Work out the finished part from the listing and answer in its coordinate system (mm). Round coordinates to 2 decimals unless told otherwise and drop trailing zeros. Order: outer loops, then holes, each group sorted by start corner. A loop starts at its lowest first (then second) coordinate and runs counter-clockwise, first axis right, second up. Notation, with made-up numbers: (57, 58) -> (83, 58) arc R21 ccw to (83, 62) -> close; hole circle Ø5 at (-1.5, 24.5). An arc over 180 degrees is marked (long way). Use one line per item in the form item = value.
```python
from build123d import *

# Parameters (mm, degrees)
SKETCH1_W           = 84.7
SKETCH1_H           = 44.8
BOSS_EXTRUDE1_DEPTH = 10.22
SKETCH2_W           = 24.5
SKETCH2_H           = 16.3
BOSS_EXTRUDE2_DEPTH = 2
SKETCH3_W           = 5.34
SKETCH3_H           = 9.1
SKETCH3_H_2         = 11.9
SKETCH3_H_3         = 11.1
SKETCH3_H_4         = 15.17
SKETCH3_H_5         = 17.32
SKETCH3_H_6         = 8
SKETCH3_H_7         = 13
SKETCH3_H_8         = 17.2
CUT_EXTRUDE1_DEPTH  = 2
SKETCH4_R           = 1.25
CUT_EXTRUDE2_DEPTH  = 50.443006583
SKETCH5_R           = 2
CUT_EXTRUDE3_DEPTH  = 1
SKETCH7_W           = 8.64
SKETCH7_H           = 3.2
CUT_EXTRUDE5_DEPTH  = 2
SKETCH8_W           = 5
SKETCH8_H           = 2
CUT_EXTRUDE6_DEPTH  = 2
SKETCH9_W           = 20.33
SKETCH9_H           = 3.1
SKETCH9_W_2         = 5.5
SKETCH9_H_2         = 2
CUT_EXTRUDE7_DEPTH  = 2
SKETCH10_W          = 13.9
SKETCH10_H          = 2.2
CUT_EXTRUDE8_DEPTH  = 2
CUT_EXTRUDE9_DEPTH  = 0.1


with BuildPart() as part:
    # Sketch1 → Boss-Extrude1 (new body)
    with BuildSketch(Plane(origin=(0, 0, 0), x_dir=(1, 0, 0), z_dir=(0, 1, 0))):
        Rectangle(SKETCH1_W, SKETCH1_H)
    extrude(amount=BOSS_EXTRUDE1_DEPTH)

    # Sketch2 → Boss-Extrude2 (add)
    with BuildSketch(Plane(origin=(0, 10.22, 0), x_dir=(1, 0, 0), z_dir=(0, 1, 0))):
        with Locations((-30.1, 0)):
            Rectangle(SKETCH2_W, SKETCH2_H)
    extrude(amount=BOSS_EXTRUDE2_DEPTH)

    # Sketch3 → Cut-Extrude1 (cut)
    with BuildSketch(Plane(origin=(0, 10.22, 0), x_dir=(1, 0, 0), z_dir=(0, 1, 0))):
        with Locations((-2.92, -15.5)):
            Rectangle(SKETCH3_W, SKETCH3_H)
        with Locations((-2.92, -1.82)):
            Rectangle(SKETCH3_W, SKETCH3_H_2)
        with Locations((-2.92, 13.95)):
            Rectangle(SKETCH3_W, SKETCH3_H_2)
        with Locations((5.22, 14.35)):
            Rectangle(SKETCH3_W, SKETCH3_H_3)
        with Locations((5.22, -1.82)):
            Rectangle(SKETCH3_W, SKETCH3_H_2)
        with Locations((5.22, -15.5)):
            Rectangle(SKETCH3_W, SKETCH3_H)
        with Locations((13.46, -15.5)):
            Rectangle(SKETCH3_W, SKETCH3_H)
        with Locations((13.46, -3.22)):
            Rectangle(SKETCH3_W, SKETCH3_H)
        with Locations((13.46, 12.315)):
            Rectangle(SKETCH3_W, SKETCH3_H_4)
        with Locations((21.6, 11.24)):
            Rectangle(SKETCH3_W, SKETCH3_H_5)
        with Locations((21.6, -4.84)):
            Rectangle(SKETCH3_W, SKETCH3_H_6)
        with Locations((21.6, -16.05)):
            Rectangle(SKETCH3_W, SKETCH3_H_6)
        with Locations((29.24, 0.8)):
            Rectangle(SKETCH3_W, SKETCH3_H_7)
        with Locations((36.88, 11.3)):
            Rectangle(SKETCH3_W, SKETCH3_H_8)
        with Locations((36.88, -11.45)):
            Rectangle(SKETCH3_W, SKETCH3_H_8)
        with Locations((-37.74, -14.1)):
            Rectangle(SKETCH3_W, SKETCH3_H_2)
        with Locations((-23.15, -14.1)):
            Rectangle(SKETCH3_W, SKETCH3_H_2)
    extrude(amount=-CUT_EXTRUDE1_DEPTH, mode=Mode.SUBTRACT)

    # Sketch4 → Cut-Extrude2 (cut, through all)
    with BuildSketch(Plane.XZ):
        with Locations(Location((-30.35, 15.75, 0), (0, 0, 270))):
            Circle(SKETCH4_R)
        with Locations(Location((-30.35, -15.75, 0), (0, 0, 270))):
            Circle(SKETCH4_R)
        with Locations(Location((31.25, 15.75, 0), (0, 0, 270))):
            Circle(SKETCH4_R)
        with Locations(Location((31.25, -15.75, 0), (0, 0, 270))):
            Circle(SKETCH4_R)
    extrude(amount=-CUT_EXTRUDE2_DEPTH, mode=Mode.SUBTRACT)

    # Sketch5 → Cut-Extrude3 (cut)
    with BuildSketch(Plane(origin=(0, 10.22, 0), x_dir=(1, 0, 0), z_dir=(0, 1, 0))):
        with Locations(Location((-30.35, -15.75, 0), (0, 0, 270))):
            Circle(SKETCH5_R)
        with Locations(Location((31.25, 15.75, 0), (0, 0, 270))):
            Circle(SKETCH5_R)
        with Locations(Location((31.25, -15.75, 0), (0, 0, 270))):
            Circle(SKETCH5_R)
        with Locations(Location((-30.35, 15.75, 0), (0, 0, 270))):
            Circle(SKETCH5_R)
    extrude(amount=-CUT_EXTRUDE3_DEPTH, mode=Mode.SUBTRACT)

    # Sketch7 → Cut-Extrude5 (cut)
    with BuildSketch(Plane.XY.offset(22.4)):
        with Locations((-11.48, 6.52)):
            Rectangle(SKETCH7_W, SKETCH7_H)
    extrude(amount=-CUT_EXTRUDE5_DEPTH, mode=Mode.SUBTRACT)

    # Sketch8 → Cut-Extrude6 (cut)
    with BuildSketch(Plane.XY.offset(22.4)):
        with Locations((23.75, 3.72)):
            Rectangle(SKETCH8_W, SKETCH8_H)
    extrude(amount=-CUT_EXTRUDE6_DEPTH, mode=Mode.SUBTRACT)

    # Sketch9 → Cut-Extrude7 (cut)
    with BuildSketch(Plane(origin=(0, 0, -22.4), x_dir=(-1, 0, 0), z_dir=(0, 0, -1))):
        with Locations((-2.885, 3.3)):
            Rectangle(SKETCH9_W, SKETCH9_H)
        with Locations((-23.2, 3.72)):
            Rectangle(SKETCH9_W_2, SKETCH9_H_2)
    extrude(amount=-CUT_EXTRUDE7_DEPTH, mode=Mode.SUBTRACT)

    # Sketch10 → Cut-Extrude8 (cut)
    with BuildSketch(Plane(origin=(42.35, 0, 0), x_dir=(0, 0, -1), z_dir=(1, 0, 0))):
        with Locations((-1.25, 3.66)):
            Rectangle(SKETCH10_W, SKETCH10_H)
    extrude(amount=-CUT_EXTRUDE8_DEPTH, mode=Mode.SUBTRACT)

    # Sketch11 → Cut-Extrude9 (cut)
    with BuildSketch(Plane(origin=(0, 12.22, 0), x_dir=(1, 0, 0), z_dir=(0, 1, 0))):
        with BuildLine():
            Line((-36.282417149, 0), (-26.882417149, 2.15))
            Line((-26.882417149, 2.15), (-27.617159632, 1.392199815))
            ThreePointArc((-27.617159632, 1.392199815), (-28.181269776, 0), (-27.617159632, -1.392199815))
            Line((-27.617159632, -1.392199815), (-26.882417149, -2.15))
            Line((-26.882417149, -2.15), (-36.282417149, 0))
        make_face()
    extrude(amount=-CUT_EXTRUDE9_DEPTH, mode=Mode.SUBTRACT)


solid = part.part
```
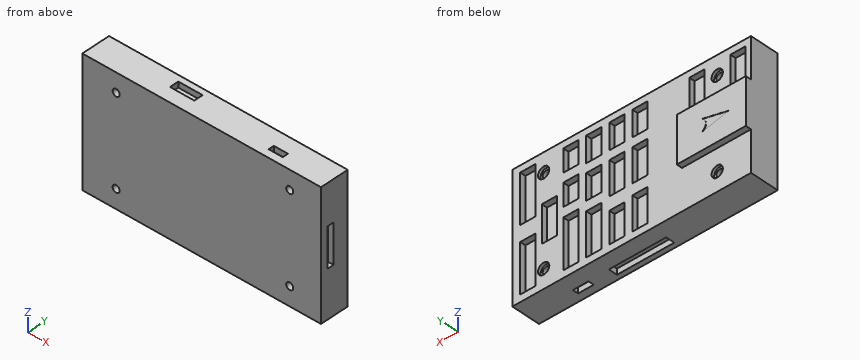
Item 1: The part is cut by section D-D, the plane x = -8.5. Give the vertices of the cut face in (y, z).
Findings:
outline = (0, -22.4) -> (10.22, -22.4) -> (10.22, 22.4) -> (8.12, 22.4) -> (8.12, 20.4) -> (4.92, 20.4) -> (4.92, 22.4) -> (0, 22.4) -> close
Item 2: The part is cut by section B-B, the plane x = -30.35. Give the vertices of the cut face in (y, z), and give its area (3 significant figures).
Findings:
outline = (0, -22.4) -> (10.22, -22.4) -> (10.22, -17.75) -> (9.22, -17.75) -> (9.22, -17) -> (0, -17) -> close; (0, -14.5) -> (9.22, -14.5) -> (9.22, -13.75) -> (10.22, -13.75) -> (10.22, -8.15) -> (12.22, -8.15) -> (12.22, -1.36) -> (12.12, -1.36) -> (12.12, 1.36) -> (12.22, 1.36) -> (12.22, 8.15) -> (10.22, 8.15) -> (10.22, 13.75) -> (9.22, 13.75) -> (9.22, 14.5) -> (0, 14.5) -> close; (0, 17) -> (9.22, 17) -> (9.22, 17.75) -> (10.22, 17.75) -> (10.22, 22.4) -> (0, 22.4) -> close
area = 436 mm^2
Item 3: The part is cut by section C-C, the plane z = -15.75. Give the number of separate pieces and of enclosed holes in the cut face, and give its area (3 significant figures).
Findings:
separate_pieces = 3
enclosed_holes = 0
area = 758 mm^2
Item 4: Consider line 1 along X through (y, z) = (5, 15.75); line 2 along X through (y, z) = (10, 8.5); line 3 along X through (y, z) = (9.5, -3.5). Determine where each line is inside the solid, lowest interval first.
Findings:
line_1 = -42.35 to -31.6, -29.1 to 30, 32.5 to 42.35
line_2 = -42.35 to -40.41, -35.07 to -25.82, -20.48 to 18.93, 24.27 to 34.21, 39.55 to 42.35
line_3 = -42.35 to -5.59, -0.25 to 2.55, 7.89 to 18.93, 24.27 to 26.57, 31.91 to 34.21, 39.55 to 42.35
Item 5: Flat-ended cylindrical pins translate along their axes: P1, Ø6, axis at x = 6.5, z = 16, coming from the +Y side; P2, Ø2.5, axis at x = 36, z = -10, coming from the +Y side. Find the tip coordinate at first contact, or state that the pin passes through.
Findings:
P1 = 10.22
P2 = 8.22
